Geometry check sheet. Reference: the model listing, model coordinates, mm. A direction names the side the tool comes from. Give positions to 0.01 mm unless a question says otherwise; leave off trailing zeros. Order: outer loops, then holes, each group sorted by start corner. A loop starts at its lowest first (then second) coordinate and runs counter-clockwise, first axis right, second up.
```python
from build123d import *

# Parameters (mm, degrees)
SKETCH1_W           = 110
SKETCH1_H           = 70
BOSS_EXTRUDE1_DEPTH = 10
SKETCH2_W           = 29
SKETCH2_H           = 29
SKETCH2_W_2         = 32
SKETCH2_H_2         = 32
SKETCH2_W_3         = 15
CUT_EXTRUDE1_DEPTH  = 8
CUT_EXTRUDE3_DEPTH  = 8
SKETCH4_R           = 1.5
CUT_EXTRUDE4_DEPTH  = 2.5
SKETCH5_W           = 46
SKETCH5_H           = 0.5
CUT_EXTRUDE5_DEPTH  = 11
SKETCH7_W           = 18
SKETCH7_H           = 2
BOSS_EXTRUDE2_DEPTH = 3


with BuildPart() as part:
    # Sketch1 → Boss-Extrude1 (new body)
    with BuildSketch(Plane.XY):
        Rectangle(SKETCH1_W, SKETCH1_H)
    extrude(amount=BOSS_EXTRUDE1_DEPTH)

    # Sketch2 → Cut-Extrude1 (cut)
    with BuildSketch(Plane.XY.offset(10)):
        with Locations((-37.5, 17.5)):
            Rectangle(SKETCH2_W, SKETCH2_H)
        with Locations((-36, -16)):
            Rectangle(SKETCH2_W_2, SKETCH2_H_2)
        with Locations((-12.5, 17.5)):
            Rectangle(SKETCH2_W_3, SKETCH2_H)
    extrude(amount=-CUT_EXTRUDE1_DEPTH, mode=Mode.SUBTRACT)

    # Sketch3 → Cut-Extrude3 (cut)
    with BuildSketch(Plane.XY.offset(10)):
        Polygon((-17, 0), (-17, -32), (52, -32), (52, 32), (-2, 32), (-2, 0), align=None)
    extrude(amount=-CUT_EXTRUDE3_DEPTH, mode=Mode.SUBTRACT)

    # Sketch4 → Cut-Extrude4 (cut)
    with BuildSketch(Plane.ZY.offset(55)):
        with Locations((5, 32)):
            Circle(SKETCH4_R)
    cut_extrude4 = extrude(amount=-CUT_EXTRUDE4_DEPTH, mode=Mode.SUBTRACT)

    # Mirror1: Cut-Extrude4 across plane
    add(cut_extrude4.mirror(Plane.ZY), mode=Mode.SUBTRACT)

    # Sketch5 → Cut-Extrude5 (cut, through all)
    with BuildSketch(Plane.XY.offset(10)):
        with Locations((-32, -34.75)):
            Rectangle(SKETCH5_W, SKETCH5_H)
        with Locations((32, -34.75)):
            Rectangle(SKETCH5_W, SKETCH5_H)
    extrude(amount=-CUT_EXTRUDE5_DEPTH, mode=Mode.SUBTRACT)

    # Sketch7 → Boss-Extrude2 (add)
    with BuildSketch(Plane.XZ.offset(35)):
        with Locations((0, 1)):
            Rectangle(SKETCH7_W, SKETCH7_H)
    extrude(amount=BOSS_EXTRUDE2_DEPTH)


solid = part.part
```
Q1. Release check for a two-part mould opening along X. For faces 4 (the face through (-36, -16, 2)), 5 (the face through (9, -34.8, 2.8)), 6 (the face through (-53.77, 30.67, 5.69)) record: pulls with the +X half, pulls with the -X half, needs draft (parallel to the pull), parting line crosses it, or undercut.
Q2. Access from +Z, -Z, +X, -X, +Y, -Y to the whole of each face (thin tool, end or side, straight path). Record for faces 1 (the face through (-20, -16, 6)), 2 (the face through (-32, -34.5, 5)), 3 (the face through (0, -35, 6)).
Q3. Cross-section at B-B, the plane x = 17.5. Record the boundary of the cut face in (y, z), and give its area (3 significant figures).
Q4. Cross-section at A-A, the plane z = 5. Give the number of separate pieces and of enclosed holes in the cut face, and give its area (3 significant figures).
Q5. Thickness scan on L1, parallel to X at y = -18, z = 4.5; L2, parallel to Y at x = -43, z = 8.5; L3, parallel to Y at x = -7, z = 3. Record the ranges inside material, lowest first.
Q6. Cross-section at D-D, the plane y = -5.5. Record the boundary of the cut face in (x, z), and give its area (3 significant figures).
Q7. Gauge pin test, flat ends, axial feed: P1, Ø2, axis at x = 1, z = 7.5, coming from the -Y side; P2, Ø1.5, axis at x = 31.5, y = -8.5, coming from the +Z side. Record the tip position at first contact, or that the pin passes through.
Q8. Cross-section at C-C, the plane y = 15. Record the boundary of the cut face in (x, z), and give its area (3 significant figures).
Answers follow:
1. face 4: undercut
1. face 5: pulls with the +X half
1. face 6: needs draft
2. face 1: +Z
2. face 2: +Z, -Z, -X, -Y
2. face 3: +Z, +X, -X, -Y
3. outline: (-34.5, 0) - (35, 0) - (35, 10) - (32, 10) - (32, 2) - (-32, 2) - (-32, 10) - (-34.5, 10) - close
3. area: 183 mm2
4. separate pieces: 1
4. enclosed holes: 4
4. area: 1,400 mm2
5. L1: x = -55 to -52, -20 to -17, 52 to 55
5. L2: y = -34.5 to -32, 0 to 3, 32 to 35
5. L3: y = -35 to -32, 0 to 3, 32 to 35
6. outline: (-55, 0) - (55, 0) - (55, 10) - (52, 10) - (52, 2) - (-17, 2) - (-17, 10) - (-20, 10) - (-20, 2) - (-52, 2) - (-52, 10) - (-55, 10) - close
6. area: 292 mm2
7. P1: stops at y = -35
7. P2: stops at z = 2
8. outline: (-55, 0) - (55, 0) - (55, 10) - (52, 10) - (52, 2) - (-2, 2) - (-2, 10) - (-5, 10) - (-5, 2) - (-20, 2) - (-20, 10) - (-23, 10) - (-23, 2) - (-52, 2) - (-52, 10) - (-55, 10) - close
8. area: 316 mm2
